from build123d import *

# Parameters (mm, degrees)
F0_R     = 3
F0_R_2   = 2.5
F1_DEPTH = 1500
F2_R     = 2
F3_R     = 7


# Not quite as in the source:
# - a feature names something its author has since deleted; it is built from what else it names


with BuildPart() as f1:
    # F0 (on Top) → F1 (new body)
    with BuildSketch(Plane.XY):
        with BuildLine():
            Line((18.15, -30), (30, -30))
            Line((30, -30), (30, -18.15))
            Line((30, -18.15), (27.5, -18.15))
            Line((27.5, -18.15), (27.5, -20.15))
            Line((27.5, -20.15), (21.5477069044, -20.15))
            ThreePointArc((21.5477069044, -20.15), (19.5, -15), (21.5477069044, -9.85))
            Line((21.5477069044, -9.85), (27.5, -9.85))
            Line((27.5, -9.85), (27.5, -11.85))
            Line((27.5, -11.85), (30, -11.85))
            Line((30, -11.85), (30, 11.85))
            Line((30, 11.85), (27.5, 11.85))
            Line((27.5, 11.85), (27.5, 9.85))
            Line((27.5, 9.85), (21.5477069044, 9.85))
            ThreePointArc((21.5477069044, 9.85), (19.5, 15), (21.5477069044, 20.15))
            Line((21.5477069044, 20.15), (27.5, 20.15))
            Line((27.5, 20.15), (27.5, 18.15))
            Line((27.5, 18.15), (30, 18.15))
            Line((30, 18.15), (30, 30))
            Line((30, 30), (18.15, 30))
            Line((18.15, 30), (18.15, 27.5))
            Line((18.15, 27.5), (20.15, 27.5))
            Line((20.15, 27.5), (20.15, 21.5477069044))
            ThreePointArc((20.15, 21.5477069044), (15, 19.5), (9.85, 21.5477069044))
            Line((9.85, 21.5477069044), (9.85, 27.5))
            Line((9.85, 27.5), (11.85, 27.5))
            Line((11.85, 27.5), (11.85, 30))
            Line((11.85, 30), (-11.85, 30))
            Line((-11.85, 30), (-11.85, 27.5))
            Line((-11.85, 27.5), (-9.85, 27.5))
            Line((-9.85, 27.5), (-9.85, 21.5477069044))
            ThreePointArc((-9.85, 21.5477069044), (-15, 19.5), (-20.15, 21.5477069044))
            Line((-20.15, 21.5477069044), (-20.15, 27.5))
            Line((-20.15, 27.5), (-18.15, 27.5))
            Line((-18.15, 27.5), (-18.15, 30))
            Line((-18.15, 30), (-30, 30))
            Line((-30, 30), (-30, 18.15))
            Line((-30, 18.15), (-27.5, 18.15))
            Line((-27.5, 18.15), (-27.5, 20.15))
            Line((-27.5, 20.15), (-21.5477069044, 20.15))
            ThreePointArc((-21.5477069044, 20.15), (-19.5, 15), (-21.5477069044, 9.85))
            Line((-21.5477069044, 9.85), (-27.5, 9.85))
            Line((-27.5, 9.85), (-27.5, 11.85))
            Line((-27.5, 11.85), (-30, 11.85))
            Line((-30, 11.85), (-30, -11.85))
            Line((-30, -11.85), (-27.5, -11.85))
            Line((-27.5, -11.85), (-27.5, -9.85))
            Line((-27.5, -9.85), (-21.5477069044, -9.85))
            ThreePointArc((-21.5477069044, -9.85), (-19.5, -15), (-21.5477069044, -20.15))
            Line((-21.5477069044, -20.15), (-27.5, -20.15))
            Line((-27.5, -20.15), (-27.5, -18.15))
            Line((-27.5, -18.15), (-30, -18.15))
            Line((-30, -18.15), (-30, -30))
            Line((-30, -30), (-18.15, -30))
            Line((-18.15, -30), (-18.15, -27.5))
            Line((-18.15, -27.5), (-20.15, -27.5))
            Line((-20.15, -27.5), (-20.15, -21.5477069044))
            ThreePointArc((-20.15, -21.5477069044), (-15, -19.5), (-9.85, -21.5477069044))
            Line((-9.85, -21.5477069044), (-9.85, -27.5))
            Line((-9.85, -27.5), (-11.85, -27.5))
            Line((-11.85, -27.5), (-11.85, -30))
            Line((-11.85, -30), (11.85, -30))
            Line((11.85, -30), (11.85, -27.5))
            Line((11.85, -27.5), (9.85, -27.5))
            Line((9.85, -27.5), (9.85, -21.5477069044))
            ThreePointArc((9.85, -21.5477069044), (15, -19.5), (20.15, -21.5477069044))
            Line((20.15, -21.5477069044), (20.15, -27.5))
            Line((20.15, -27.5), (18.15, -27.5))
            Line((18.15, -27.5), (18.15, -30))
        make_face()
        with Locations((-25, -25)):
            Circle(F0_R, mode=Mode.SUBTRACT)
        with Locations((-15, -15)):
            Circle(F0_R_2, mode=Mode.SUBTRACT)
        with Locations((25, -25)):
            Circle(F0_R, mode=Mode.SUBTRACT)
        with Locations((15, -15)):
            Circle(F0_R_2, mode=Mode.SUBTRACT)
        with Locations((-25, 25)):
            Circle(F0_R, mode=Mode.SUBTRACT)
        with Locations((-15, 15)):
            Circle(F0_R_2, mode=Mode.SUBTRACT)
        Polygon((-7, 22), (-7, 27.5), (0, 27.5), (7, 27.5), (7, 22), (10, 16), (10, 10), (16, 10), (22, 7), (27.5, 7), (27.5, 0), (27.5, -7), (22, -7), (16, -10), (10, -10), (10, -16), (7, -22), (7, -27.5), (0, -27.5), (-7, -27.5), (-7, -22), (-10, -16), (-10, -10), (-16, -10), (-22, -7), (-27.5, -7), (-27.5, 0), (-27.5, 7), (-22, 7), (-16, 10), (-10, 10), (-10, 16), align=None, mode=Mode.SUBTRACT)
        with Locations((15, 15)):
            Circle(F0_R_2, mode=Mode.SUBTRACT)
        with Locations((25, 25)):
            Circle(F0_R, mode=Mode.SUBTRACT)
    extrude(amount=F1_DEPTH)

    # F2
    f2_edges = [f1.edges().sort_by_distance(p)[0] for p in [
        (-7, 27.5, 750),
        (7, 27.5, 750),
    ]]
    fillet(f2_edges, radius=F2_R)

    # F3
    f3_edges = [f1.edges().sort_by_distance(p)[0] for p in [
        (-10, 16, 750),
        (10, 16, 750),
    ]]
    fillet(f3_edges, radius=F3_R)


solid = f1.part
Design review of the part built by this model. Coordinates are the model's own, in mm. Give positions to 0.01 mm unless a question says otherwise; leave off trailing zeros.
1. For pin 1 Ø3 at (y, z) = (-14.5, 984.5) entering from -X, flat-tipped, find the tip position at first contact; note if it passes through.
Solution:
pin 1: stops at x = -19.77
2. To check wall thickness, follow L1, parallel to Y at x = -14.5, z = 710.5; L2, parallel to X at y = -26, z = 1284; L3, parallel to Y at x = -15, z = 752. State the ranges of each line that lie inside material, in increasing order.
Solution:
L1: y = -19.52 to -17.45, -12.55 to -10, 10 to 12.55, 17.45 to 19.52
L2: x = -30 to -27.83, -22.17 to -20.15, -9.85 to -7, 7 to 9.85, 20.15 to 22.17, 27.83 to 30
L3: y = -19.5 to -17.5, -12.5 to -10, 10 to 12.5, 17.5 to 19.5
3. Add section A-A, the plane z = 527. State how many separate pieces and enclosed holes the cut face has, then the cut area to 3 significant figures.
Solution:
separate pieces: 1
enclosed holes: 9
area: 1,080 mm2
